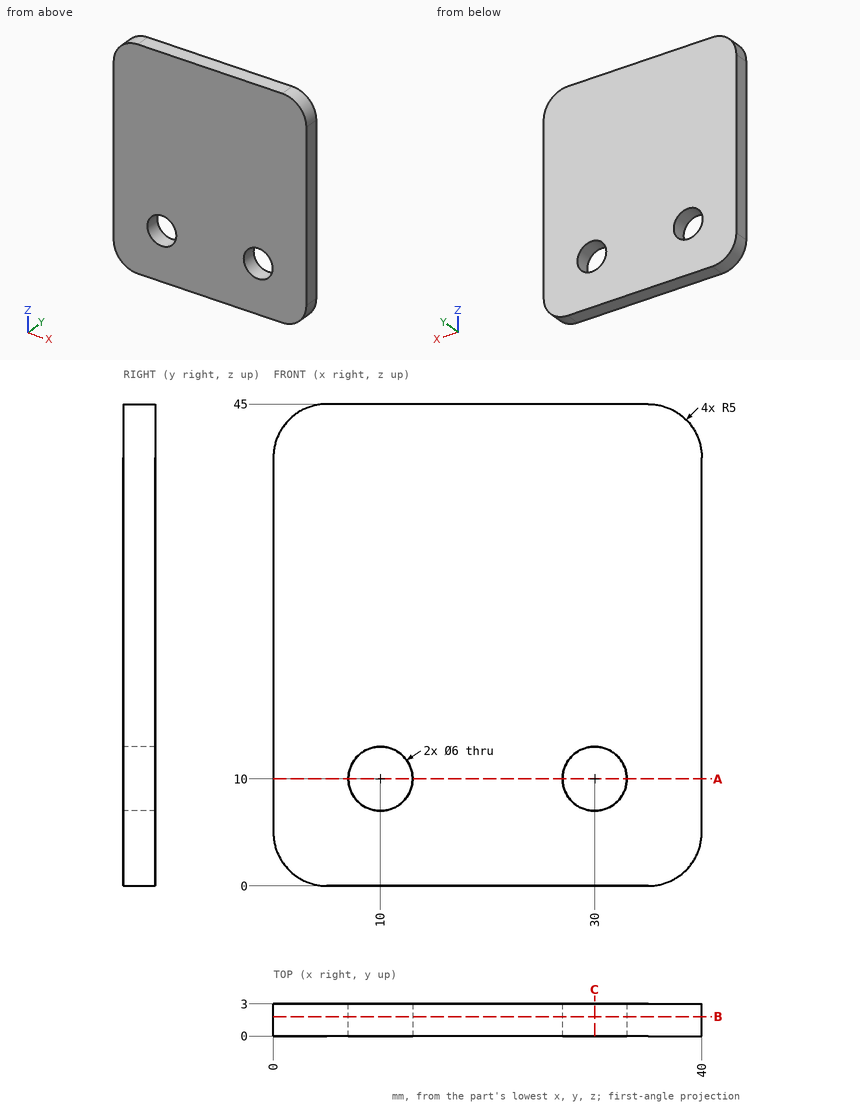
Geometry: see drawing. Coordinates: mm, zero at the bounding-box minimum. Give positions to 0.01 mm unless a question says otherwise; leave off trailing zeros. Order: outer loops, then holes, each group sorted by start corner. A loop starts at its lowest first (then second) coordinate and runs counter-clockwise, first axis right, second up. Notation, with made-up numbers: M 72,-31 L 119,-31 A25 ccw 119,4 Z; hole C 24.5,21 d4. An arc over 180 degrees is marked long. Answer as CSV lines item,"result". Start each with the question number.
1) Cut plane C-C (x = 30). Output: boundary loops of the cut face in (y, z).
2) Line query: line 1 (X direction, y = 1.9, z = 10); line 2 (Z direction, x = 10, y = 0.35); line 3 (X direction, y = 2.7, z = 7.5). Output: solid intervals per line, ascending. Write a range as from..to.
3) Cut plane A-A (z = 10). Output: boundary loops of the cut face in (x, y).
4) First-contact query: P1, Ø3.5, axis at x = 10, z = 10, coming from the +Y side. Flat tip, straight axial feed; report the tip coordinate or a pass-through.
5) Cut plane B-B (y = 1.8). Output: boundary loops of the cut face in (x, z), then the cut area to 3 significant figures.
Findings below:
1,outline,"M 0,0 L 3,0 L 3,7 L 0,7 Z; M 0,13 L 3,13 L 3,45 L 0,45 Z"
2,line 1,"x = 0..7, 13..27, 33..40"
2,line 2,"z = 0..7, 13..45"
2,line 3,"x = 0..8.34, 11.66..28.34, 31.66..40"
3,outline,"M 0,0 L 7,0 L 7,3 L 0,3 Z; M 13,0 L 27,0 L 27,3 L 13,3 Z; M 33,0 L 40,0 L 40,3 L 33,3 Z"
4,P1,"passes through"
5,outline,"M 0,5 A5 ccw 5,0 L 35,0 A5 ccw 40,5 L 40,40 A5 ccw 35,45 L 5,45 A5 ccw 0,40 Z; hole C 10,10 d6; hole C 30,10 d6"
5,area,"1,720 mm²"
